```python
from build123d import *

# Parameters (mm, degrees)
SKETCH046_W             = 102
SKETCH046_H             = 146
PAD012_DEPTH            = 26
SKETCH047_R             = 2
POCKET033_DEPTH         = 102.001
CHAMFER001_SIZE         = 2
BODY010_PLACEMENT_ANGLE = 180


with BuildPart() as part:
    # Sketch046 → Pad012 (new body)
    with BuildSketch(Plane.XY):
        Rectangle(SKETCH046_W, SKETCH046_H)
    extrude(amount=PAD012_DEPTH)

    # Sketch047 (on Face3 of Pad012) → Pocket033 (cut, through all)
    with BuildSketch(Plane.YZ.offset(51)):
        with Locations((45, 6)):
            Circle(SKETCH047_R)
        with Locations((3.4, 6)):
            Circle(SKETCH047_R)
        with Locations((-56.6, 6)):
            Circle(SKETCH047_R)
    extrude(amount=-POCKET033_DEPTH, mode=Mode.SUBTRACT)

    # Chamfer001
    chamfer001_edges = [part.edges().sort_by_distance(p)[0] for p in [
        (-51, 0, 0),
        (0, -73, 0),
        (51, 0, 0),
        (0, 73, 0),
        (-51, 0, 26),
        (0, -73, 26),
        (51, 0, 26),
        (0, 73, 26),
    ]]
    chamfer(chamfer001_edges, length=CHAMFER001_SIZE)


with BuildPart() as part_1:
    # Body010 placement: moved
    add(part.part.moved(Location((63.5, 58.3, 8))).rotate(Axis((63.5, 58.3, 8), (0, 0, 1)), BODY010_PLACEMENT_ANGLE))


solid = part_1.part
```
Check sheet for the modelled part. Datum: model origin and axes. Units: mm. Coordinates: 2 decimals unless noted, no trailing zeros. Loops run counter-clockwise (first coordinate to the right, second up) from the corner with the lowest first, then second, coordinate; pieces in that order, holes last.
1) Release check for a two-part mould opening along Y. For faces 1 (the face through (64, 131.3, 21)), 2 (the face through (64, 57, 34)), 3 (the face through (62.786, 56.898, 14.088)) record: released by +Y, released by -Y, zero draft, split by the parting line, or undercut.
2) Sectioned sample at B-B (z = 14). Record the boundary of the cut face in (x, y).
3) Material ranges on probe 1 along Z at (x, y) = (72, 13.3); probe 2 along Y at (x, z) = (73, 13.5); probe 3 along Z at (x, y) = (73, 54), recorded low to high.
4) Sectioned sample at A-A (y = 13.3). Record the boundary of the cut face in (x, z), and give its area (3 significant figures).
Check sheet entries:
1. face 1: released by +Y
1. face 2: zero draft
1. face 3: undercut
2. outline: (12.5, -14.7) - (114.5, -14.7) - (114.5, 11.3) - (12.5, 11.3) - close; (12.5, 15.3) - (114.5, 15.3) - (114.5, 52.9) - (12.5, 52.9) - close; (12.5, 56.9) - (114.5, 56.9) - (114.5, 112.9) - (12.5, 112.9) - close; (12.5, 116.9) - (114.5, 116.9) - (114.5, 131.3) - (12.5, 131.3) - close
3. probe 1: z = 8 to 12, 16 to 34
3. probe 2: y = -14.7 to 11.36, 15.24 to 52.96, 56.84 to 112.96, 116.84 to 131.3
3. probe 3: z = 8 to 12.21, 15.79 to 34
4. outline: (12.5, 10) - (14.5, 8) - (112.5, 8) - (114.5, 10) - (114.5, 12) - (12.5, 12) - close; (12.5, 16) - (114.5, 16) - (114.5, 32) - (112.5, 34) - (14.5, 34) - (12.5, 32) - close
4. area: 2,240 mm2
